Design review of the part built by this model. Coordinates are the model's own, in mm. A direction names the side the tool comes from. Coordinates: 2 decimals unless noted, no trailing zeros. Loops run counter-clockwise (first coordinate to the right, second up) from the corner with the lowest first, then second, coordinate; pieces in that order, holes last. Notation, with made-up numbers: (4.5, -3.75) -> (49.5, -3.75) arc R13 cw to (49.5, 1.25) -> close; hole circle Ø5 at (34.5, -3). An arc over 180 degrees is marked (long way). Answer in a Markdown table with one row per item.
Autodesk Fusion 360 part; units mm, degrees
sketch "Sketch1" plane through (0, 0, 0) normal (0, 1, 0) x (1, 0, 0)
  line L0 (56.5, -34) -> (-56.5, -34)
  line L1 (-56.5, -34) -> (-56.5, 34)
  line L2 (-56.5, 34) -> (56.5, 34)
  line L3 (56.5, 34) -> (56.5, -34)
  line L4 (56.5, -34) -> (-56.5, 34) construction
  line L5 (-56.5, -34) -> (56.5, 34) construction
  line L6 (64, 30) -> (-64, 30)
  line L7 (-64, 30) -> (-64, -30)
  line L8 (-64, -30) -> (64, -30)
  line L9 (64, -30) -> (64, 30)
  line L10 (64, 30) -> (-64, -30) construction
  line L11 (-64, 30) -> (64, -30) construction
  circle A0 centre (64, 30) radius 1.25
  line L12 (60.5, -38) -> (-60.5, -38)
  line L13 (-60.5, -38) -> (-60.5, 38)
  line L14 (-60.5, 38) -> (60.5, 38)
  line L15 (60.5, 38) -> (60.5, -38)
  line L16 (60.5, -38) -> (-60.5, 38) construction
  line L17 (-60.5, -38) -> (60.5, 38) construction
  circle A1 centre (-56.5, 34) radius 1.25
  circle A2 centre (-56.5, 34) radius 3
  circle A3 centre (56.5, 34) radius 1.25
  circle A4 centre (56.5, 34) radius 3
  circle A5 centre (56.5, -34) radius 1.25
  circle A6 centre (56.5, -34) radius 3
  circle A7 centre (-56.5, -34) radius 1.25
  circle A8 centre (-56.5, -34) radius 3
  circle A9 centre (64, -30) radius 1.25
  circle A10 centre (-64, -30) radius 1.25
  circle A11 centre (-64, 30) radius 1.25
  circle A12 centre (-64, 30) radius 3
  circle A13 centre (64, 30) radius 3
  circle A14 centre (64, -30) radius 3
  circle A15 centre (-64, -30) radius 3
  line L18 (61, -38.5) -> (-61, -38.5)
  line L19 (-61, -38.5) -> (-61, 38.5)
  line L20 (-61, 38.5) -> (61, 38.5)
  line L21 (61, 38.5) -> (61, -38.5)
  line L22 (61, -38.5) -> (-61, 38.5) construction
  line L23 (-61, -38.5) -> (61, 38.5) construction
  line L24 (67.5, -42.5) -> (-67.5, -42.5)
  line L25 (-67.5, -42.5) -> (-67.5, 42.5)
  line L26 (-67.5, 42.5) -> (67.5, 42.5)
  line L27 (67.5, 42.5) -> (67.5, -42.5)
  line L28 (67.5, -42.5) -> (-67.5, 42.5) construction
  line L29 (-67.5, -42.5) -> (67.5, 42.5) construction
  dimension "d1" = 113
  dimension "d2" = 68
  dimension "d3" = 128
  dimension "d4" = 60
  dimension "d5" = 2.5
  dimension "d6" = 121
  dimension "d7" = 76
  dimension "d8" = 2.5
  dimension "d9" = 6
  dimension "d10" = 2.5
  dimension "d11" = 6
  dimension "d12" = 2.5
  dimension "d13" = 6
  dimension "d14" = 2.5
  dimension "d15" = 6
  dimension "d16" = 2.5
  dimension "d17" = 2.5
  dimension "d18" = 2.5
  dimension "d19" = 6
  dimension "d20" = 6
  dimension "d21" = 6
  dimension "d22" = 6
  dimension "d25" = 122
  dimension "d26" = 77
  dimension "d27" = 135
  dimension "d28" = 85
extrude "Extrude1" add sketch "Sketch1" along normal blind 8 contours L0 L1 A7 A8 | L0 L1 A7 A8 | L0 L3 A5 A6 | L0 L3 A5 A6 | L1 L2 A1 A2 | L1 L2 A1 A2 | L2 L3 A3 A4 | L2 L3 A3 A4 makes body 1 at (-53.5149, 5.3333, -34.2987) makes body 2 at (-53.5149, 2.6667, 33.7013) makes body 3 at (59.4851, 2.6667, -34.2987) makes body 4 at (59.4851, 2.6667, 33.7013)
extrude "Extrude2" add sketch "Sketch1" along normal blind 15 separate body contours L7 A12 A15 L19 | L9 A13 A14 L21 | L24 L25 L26 L27 makes body 5
extrude "Extrude3" add sketch "Sketch1" along normal blind 10 separate body contours L7 L8 A10 A15 | L7 L8 A10 A15 | L8 L9 A9 A14 | L8 L9 A9 A14 | L6 L7 A11 A12 | L6 L7 A11 A12 | L6 L9 A0 A13 | L6 L9 A0 A13 makes body 6 at (64.5209, 6.6667, 32.9544) makes body 7 at (-61.0149, 6.6667, 29.7013) makes body 8 at (64.9555, 3.3333, -32.8438) makes body 9 at (-61.0149, 3.3333, -30.2987)
sketch "Sketch2" plane through (0, 15, 0) normal (0, 1, 0) x (-1, 0, 0)
  line L0 (61, -38.5) -> (-61, -38.5)
  line L1 (-61, -38.5) -> (-61, -30)
  circle A0 centre (-64, -30) radius 3
  line L2 (-61, -30) -> (-61, 30)
  circle A1 centre (-64, 30) radius 3
  line L3 (-61, 30) -> (-61, 38.5)
  line L4 (-61, 38.5) -> (61, 38.5)
  line L5 (61, 38.5) -> (61, 30)
  circle A2 centre (64, 30) radius 3
  line L6 (61, 30) -> (61, -30)
  circle A3 centre (64, -30) radius 3
  line L7 (61, -30) -> (61, -38.5)
  line L8 (-67.5, -42.5) -> (67.5, -42.5)
  line L9 (67.5, -42.5) -> (67.5, 42.5)
  line L10 (67.5, 42.5) -> (-67.5, 42.5)
  line L11 (-67.5, 42.5) -> (-67.5, -42.5)
  line L12 (-56.5, -34) -> (56.5, -34)
  line L13 (56.5, -34) -> (56.5, 34)
  line L14 (56.5, 34) -> (-56.5, 34)
  line L15 (-56.5, 34) -> (-56.5, -34)
  line L16 (-56.5, -34) -> (56.5, 34) construction
  line L17 (56.5, -34) -> (-56.5, 34) construction
  circle A4 centre (56.5, -34) radius 1.25
  circle A5 centre (56.5, -34) radius 3
  line L18 (56.5, -31) -> (61, -31)
  line L19 (53.5, -34) -> (53.5, -38.5)
  line L20 (0, 0) -> (0, -46.2304) construction
  line L21 (0, 0) -> (-40.9385, 0) construction
  line L22 (-53.5, -34) -> (-53.5, -38.5)
  circle A6 centre (-56.5, -34) radius 3
  circle A7 centre (-56.5, -34) radius 1.25
  line L23 (-56.5, -31) -> (-61, -31)
  line L24 (56.5, 31) -> (61, 31)
  circle A8 centre (56.5, 34) radius 3
  circle A9 centre (56.5, 34) radius 1.25
  line L25 (53.5, 34) -> (53.5, 38.5)
  line L26 (-56.5, 31) -> (-61, 31)
  circle A10 centre (-56.5, 34) radius 3
  circle A11 centre (-56.5, 34) radius 1.25
  line L27 (-53.5, 34) -> (-53.5, 38.5)
  dimension "d33" = 113
  dimension "d34" = 68
  dimension "d35" = 2.5
  dimension "d36" = 6
extrude "Extrude4" add sketch "Sketch2" against normal blind 7 separate body contours L0 L7 A5 L18 L19 | L0 L1 L22 A6 L23 | L12 L13 A4 A5 | L12 L13 A4 A5 | L12 L15 A6 A7 | L12 L15 A6 A7 | L13 L14 A8 A9 | L4 L5 L24 A8 L25 | L13 L14 A8 A9 | L14 L15 A10 A11 | L3 L4 L26 A10 L27 | L14 L15 A10 A11 makes body 10 at (-57.4576, 12.6667, 34.8035) makes body 11 at (55.5036, 10.3333, -34.7548) makes body 12 at (57.6746, 12.6667, 33.5725) makes body 13 at (-55.3254, 10.3333, -33.5725)
combine "Combine1" operation add target body 13 tool bodies 12 11 10 5 9 8 7 6
hidden bodies 1 2 3 4
(1) Draft analysis for pull direction X (two halves, no side actions). For faces 1 (the cylindrical face through (65.19, 4.93, -29.62)), 2 (the flat face through (59, 12, -31)), 3 (the flat face through (-1, 7, -42.5)), 4 (the flat face through (-67.5, 7, 1)), state which applies: pulls with the +X half, pulls with the -X half, needs draft (parallel to the pull), parting line crosses it, or undercut.
Evaluation:
| item | result |
|---|---|
| face 1 | undercut |
| face 2 | undercut |
| face 3 | needs draft |
| face 4 | pulls with the -X half |
(2) For pin 1 (4 mm diameter, centred on x = -56, z = -34, fed in from -Y); pin 2 (12 mm diameter, centred on x = -18, z = 27, fed in from +Y); pin 3 (4 mm diameter, centred on x = -64, z = -30, fed in from +Y), all flat-tipped, find the tip position at first contact; note any pin that passes through.
Evaluation:
| item | result |
|---|---|
| pin 1 | stops at y = 8 |
| pin 2 | passes through |
| pin 3 | stops at y = 10 |
(3) Take a section at B-B on x = -11. Give the boundary of the cut face in (y, z).
Evaluation:
| item | result |
|---|---|
| outline | (0, -42.5) -> (15, -42.5) -> (15, -38.5) -> (0, -38.5) -> close; (0, 38.5) -> (15, 38.5) -> (15, 42.5) -> (0, 42.5) -> close |
(4) Take a section at A-A on y = 2.25. Give the boundary of the cut face in (x, z), and give its area (3 significant figures).
Evaluation:
| item | result |
|---|---|
| outline | (-67.5, -42.5) -> (67.5, -42.5) -> (67.5, 42.5) -> (-67.5, 42.5) -> close; hole circle Ø2.5 at (-64, -30); hole circle Ø2.5 at (-64, 30); hole (-61, -38.5) -> (61, -38.5) -> (61, 38.5) -> (-61, 38.5) -> close; hole circle Ø2.5 at (64, -30); hole circle Ø2.5 at (64, 30) |
| area | 2,060 mm² |
(5) Tool access review of faces 5 (the flat face through (67.5, 7, -1)), 6 (the flat face through (65, 10, 31)), 7 (the flat face through (-53.5, 12, 36)), 8 (the flat face through (-57, 8, 36)): name each direction out of +Z, -Z, +X, -X, +Y, -Y from which nothing blocks a thin tool from reaching the whole face with its end or side.
Evaluation:
| item | result |
|---|---|
| face 5 | +Z, -Z, +X, +Y, -Y |
| face 6 | +Y |
| face 7 | +Y, -Y |
| face 8 | -Y |
(6) Take a section at D-D on z = 37. Give the boundary of the cut face in (x, y), and give its area (3 significant figures).
Evaluation:
| item | result |
|---|---|
| outline | (-67.5, 0) -> (-61, 0) -> (-61, 8) -> (-53.5, 8) -> (-53.5, 15) -> (-67.5, 15) -> close; (53.5, 8) -> (61, 8) -> (61, 0) -> (67.5, 0) -> (67.5, 15) -> (53.5, 15) -> close |
| area | 300 mm² |
(7) To check wall thickness, follow probe 1 along Z at (x, y) = (56.5, 10.75); probe 2 along X at (y, z) = (5.75, -30); probe 3 along X at (y, z) = (10.5, 34). State the ranges of each line that lie inside material, in increasing order.
Evaluation:
| item | result |
|---|---|
| probe 1 | z = -42.5 to -35.25, -32.75 to -31, 31 to 32.75, 35.25 to 42.5 |
| probe 2 | x = -67.5 to -65.25, -62.75 to -61, 61 to 62.75, 65.25 to 67.5 |
| probe 3 | x = -67.5 to -57.75, -55.25 to -53.5, 53.5 to 55.25, 57.75 to 67.5 |
